The listing builds one solid part. Answer for the finished solid, in the listing's coordinates (mm). A direction names the side the tool comes from. Coordinates: 2 decimals unless noted, no trailing zeros. Order: outer loops, then holes, each group sorted by start corner. A loop starts at its lowest first (then second) coordinate and runs counter-clockwise, first axis right, second up. Notation, with made-up numbers: (17, -9.75) - (28, -9.75) arc R25 cw to (28, 25.25) - close; hole circle Ø6 at (78, 64.5). An arc over 180 degrees is marked (long way). One line per item, written item: value. Start each with the question number.
```python
from build123d import *

# Parameters (mm, degrees)
SKETCH1_W           = 42.164
SKETCH1_H           = 33.9852
SKETCH1_R           = 9.017
SKETCH1_R_2         = 1.0668
SKETCH1_R_3         = 1.063335115
BOSS_EXTRUDE1_DEPTH = 1


with BuildPart() as part:
    # Sketch1 → Boss-Extrude1 (new body)
    with BuildSketch(Plane(origin=(0, 0, -1.017418828), x_dir=(-1, 0, 0), z_dir=(0, 0, -1))):
        with Locations((105.86640625, -147.03953125)):
            Rectangle(SKETCH1_W, SKETCH1_H)
        with Locations((105.86640625, -141.16895625)):
            Circle(SKETCH1_R, mode=Mode.SUBTRACT)
        with Locations((92.118252965, -149.10645625)):
            Circle(SKETCH1_R_2, mode=Mode.SUBTRACT)
        with Locations((92.118252965, -133.23145625)):
            Circle(SKETCH1_R_2, mode=Mode.SUBTRACT)
        with Locations((119.614559536, -133.23145625)):
            Circle(SKETCH1_R_2, mode=Mode.SUBTRACT)
        with Locations((105.86640625, -157.04395625)):
            Circle(SKETCH1_R_2, mode=Mode.SUBTRACT)
        with Locations((115.01040625, -149.10645625)):
            Circle(SKETCH1_R_3, mode=Mode.SUBTRACT)
        with Locations((121.614405679, -159.20295625)):
            Circle(SKETCH1_R_2, mode=Mode.SUBTRACT)
        with BuildLine():
            Line((118.356545978, -137.93013125), (124.856545978, -137.93013125))
            ThreePointArc((124.856545978, -137.93013125), (125.210099369, -138.07657786), (125.356545978, -138.43013125))
            Line((125.356545978, -138.43013125), (125.356545978, -144.93013125))
            ThreePointArc((125.356545978, -144.93013125), (125.210099369, -145.283684641), (124.856545978, -145.43013125))
            Line((124.856545978, -145.43013125), (118.356545978, -145.43013125))
            ThreePointArc((118.356545978, -145.43013125), (118.002992588, -145.283684641), (117.856545978, -144.93013125))
            Line((117.856545978, -144.93013125), (117.856545978, -138.43013125))
            ThreePointArc((117.856545978, -138.43013125), (118.002992588, -138.07657786), (118.356545978, -137.93013125))
        make_face(mode=Mode.SUBTRACT)
        with BuildLine():
            Line((124.856545978, -157.36813125), (118.356545978, -157.36813125))
            ThreePointArc((118.356545978, -157.36813125), (118.002992588, -157.221684641), (117.856545978, -156.86813125))
            Line((117.856545978, -156.86813125), (117.856545978, -150.36813125))
            ThreePointArc((117.856545978, -150.36813125), (118.002992588, -150.01457786), (118.356545978, -149.86813125))
            Line((118.356545978, -149.86813125), (124.856545978, -149.86813125))
            ThreePointArc((124.856545978, -149.86813125), (125.210099369, -150.01457786), (125.356545978, -150.36813125))
            Line((125.356545978, -150.36813125), (125.356545978, -156.86813125))
            ThreePointArc((125.356545978, -156.86813125), (125.210099369, -157.221684641), (124.856545978, -157.36813125))
        make_face(mode=Mode.SUBTRACT)
    extrude(amount=-BOSS_EXTRUDE1_DEPTH)


solid = part.part
```
(1) A flat-ended cylindrical pin translates along its axis: pin 1 Ø1.9 at (x, y) = (-92.12, -149.11) entering from +Z. Find the tip coordinate at first contact, or state that the pin passes through.
(2) For a pull along Y with two mould halves and no side action, classify faces 3 (the face through (-116, -149.5, -0.5)), 4 (the face through (-126.948, -147.3, -0.5)), 5 (the face through (-105.6, -164.032, -0.5)), 6 (the face through (-121.7, -157.368, -0.5)) as pulls with the +Y half, pulls with the -Y half, needs draft (parallel to the pull), parting line crosses it, or undercut.
(3) The part is cut by section C-C on z = -0.5. Count the separate pieces of the cut face and the enclosed holes in it, plus the area to 3 significant figures.
(4) The part is cut by section A-A on y = -152.5. Determine the outline of the cut face in (x, z).
(5) The part is cut by section D-D on x = -92.5. Determine the outline of the cut face in (y, z), plus the area to 3 significant figures.
(6) For faces 1 (the face through (-106, -151, -1.017)), 2 (the face through (-121.6, -137.93, -0.5)), determine the directions among +Z, -Z, +X, -X, +Y, -Y from which every point of the face is accessible in a straight line to the end or side of a thin tool.
(7) Consider probe 1 along Y at (x, z) = (-124, -0.5); probe 2 along Y at (x, z) = (-106.5, -0.65); probe 3 along X at (y, z) = (-134, -0.2). Determine where each line is inside the solid, lowest interval first.
(8) The part is cut by section B-B on x = -109. Determine the outline of the cut face in (y, z).
Completed:
1. pin 1: passes through
2. face 3: undercut
2. face 4: needs draft
2. face 5: pulls with the -Y half
2. face 6: undercut
3. separate pieces: 1
3. enclosed holes: 9
3. area: 1,040 mm2
4. outline: (-126.95, -1.02) - (-125.36, -1.02) - (-125.36, -0.02) - (-126.95, -0.02) - close; (-117.86, -1.02) - (-84.78, -1.02) - (-84.78, -0.02) - (-117.86, -0.02) - close
5. outline: (-164.03, -1.02) - (-150.1, -1.02) - (-150.1, -0.02) - (-164.03, -0.02) - close; (-148.11, -1.02) - (-134.23, -1.02) - (-134.23, -0.02) - (-148.11, -0.02) - close; (-132.24, -1.02) - (-130.05, -1.02) - (-130.05, -0.02) - (-132.24, -0.02) - close
5. area: 30.0 mm2
6. face 1: -Z, +X, -X, +Y, -Y
6. face 2: +Z, -Z
7. probe 1: y = -164.03 to -157.37, -149.87 to -145.43, -137.93 to -130.05
7. probe 2: y = -164.03 to -157.9, -156.19 to -150.16, -132.17 to -130.05
7. probe 3: x = -126.95 to -120.35, -118.87 to -111.34, -100.4 to -92.86, -91.38 to -84.78
8. outline: (-164.03, -1.02) - (-149.62, -1.02) - (-149.62, -0.02) - (-164.03, -0.02) - close; (-132.71, -1.02) - (-130.05, -1.02) - (-130.05, -0.02) - (-132.71, -0.02) - close
